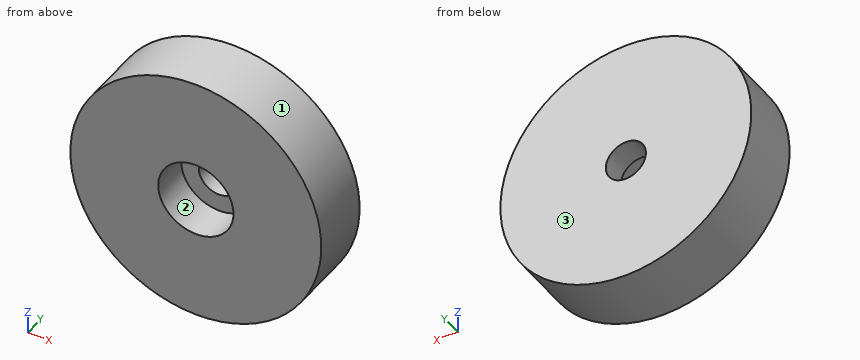
```python
from build123d import *

# Parameters (mm, degrees)
SKETCH1_R           = 10
BOSS_EXTRUDE1_DEPTH = 5
CUT_EXTRUDE1_START  = -2
SKETCH2_R           = 3
CUT_EXTRUDE1_DEPTH  = 5
SKETCH3_R           = 1.6
CUT_EXTRUDE2_DEPTH  = 16


with BuildPart() as part:
    # Sketch1 → Boss-Extrude1 (new body)
    with BuildSketch(Plane(origin=(0, 0, 0), x_dir=(1, 0, 0), z_dir=(0, 1, 0))):
        with Locations(Location((0, 0, 0), (0, 0, 270))):
            Circle(SKETCH1_R)
    extrude(amount=BOSS_EXTRUDE1_DEPTH)

    # Sketch2 → Cut-Extrude1 (cut)
    with BuildSketch(Plane(origin=(0, 5, 0), x_dir=(1, 0, 0), z_dir=(0, 1, 0)).offset(CUT_EXTRUDE1_START)):
        with Locations(Location((0, 0, 0), (0, 0, 270))):
            Circle(SKETCH2_R)
    extrude(amount=-CUT_EXTRUDE1_DEPTH, mode=Mode.SUBTRACT)

    # Sketch3 → Cut-Extrude2 (cut, through all)
    with BuildSketch(Plane(origin=(0, 5, 0), x_dir=(1, 0, 0), z_dir=(0, 1, 0))):
        with Locations(Location((0, 0, 0), (0, 0, 270))):
            Circle(SKETCH3_R)
    extrude(amount=-CUT_EXTRUDE2_DEPTH, mode=Mode.SUBTRACT)


solid = part.part
```
Read the model definition and answer for the solid it produces. Units are mm, in the model's axes. Face numbers are marked on the shaded views. Round coordinates to 2 decimals unless told otherwise and drop trailing zeros. Write each loop counter-clockwise with the first axis right and the second up, starting at its lowest first coordinate (ties: lowest second). Pieces come first, ordered by that corner, then holes. Notation, with made-up numbers: (-32.5, -9) - (3.5, -9) arc R7 cw to (3.5, -2) - close; hole circle Ø5 at (60, 60). An arc over 180 degrees is marked (long way). One line per item, written item: value.
Q1. Find section C-C (y = 3.9). Determine the outline of the cut face in (x, z), and give its area (3 significant figures).
The answers:
outline: circle Ø20 at (0, 0); hole circle Ø3.2 at (0, 0)
area: 306 mm2
Q2. Find section B-B (z = 0). Determine the outline of the cut face in (x, y), and give its area (3 significant figures).
The answers:
outline: (-10, 0) - (-3, 0) - (-3, 3) - (-1.6, 3) - (-1.6, 5) - (-10, 5) - close; (1.6, 3) - (3, 3) - (3, 0) - (10, 0) - (10, 5) - (1.6, 5) - close
area: 75.6 mm2
Q3. Find section D-D (z = 2.75). Determine the outline of the cut face in (x, y), and give its area (3 significant figures).
The answers:
outline: (-9.61, 0) - (-1.2, 0) - (-1.2, 3) - (1.2, 3) - (1.2, 0) - (9.61, 0) - (9.61, 5) - (-9.61, 5) - close
area: 89.0 mm2
Q4. Find section A-A (x = 0). Determine the outline of the cut face in (y, z), and give its area (3 significant figures).
The answers:
outline: (0, -10) - (5, -10) - (5, -1.6) - (3, -1.6) - (3, -3) - (0, -3) - close; (0, 3) - (3, 3) - (3, 1.6) - (5, 1.6) - (5, 10) - (0, 10) - close
area: 75.6 mm2
Q5. Straight lines are drawn through the part: line 1 (X direction, y = 4.05, z = 0); line 2 (X direction, y = 0.7, z = 0); line 3 (Z direction, x = 1, y = 2.9). For each, find the intervals that lie inside material, in ascending order. Write a range as from..to.
The answers:
line 1: x = -10..-1.6, 1.6..10
line 2: x = -10..-3, 3..10
line 3: z = -9.95..-2.83, 2.83..9.95
Q6. For a pull along X with two mould halves and no side action, classify the marked faces 1, 2 and 3 as pulls with the +X half, pulls with the -X half, needs draft (parallel to the pull), parting line crosses it, or undercut.
The answers:
face 1: parting line crosses it
face 2: undercut
face 3: needs draft
Q7. Each of these flat-tipped pins is pushed along its axis until it touches: P1, Ø1.5, axis at y = 1.5, z = -6.5, coming from the +X side; P2, Ø5, axis at x = 0, z = 0, coming from the -Y side; P3, Ø2, axis at y = 1.5, z = 6, coming from the -X side. Where does it stop, or does it pass through?
The answers:
P1: stops at x = 8.18
P2: stops at y = 3
P3: stops at x = -8.66
